Geometry check sheet. Reference: the model listing, model coordinates, mm. A direction names the side the tool comes from. Coordinates: 2 decimals unless noted, no trailing zeros. Write each loop counter-clockwise with the first axis right and the second up, starting at its lowest first coordinate (ties: lowest second). Pieces come first, ordered by that corner, then holes.
Autodesk Inventor part; units mm, degrees
ref_plane "Start plane" through (0, 0, 0) normal (0, 0, 1) x (1, 0, 0)
ref_plane "End plane" through (0, 0, 1263.65) normal (0, 0, 1) x (1, 0, 0)
ref_plane "Work Plane4" through (19.05, 0, 1263.65) normal (0, 0.7071, 0.7071) x (1, 0, 0)
ref_plane "Start plane" through (0, 0, 0) normal (0, 0, 1) x (1, 0, 0)
ref_plane "End plane" through (0, 0, 1263.65) normal (0, 0, 1) x (1, 0, 0)
sketch "Sketch" plane through (0, 0, 0) normal (0, 0, 1) x (1, 0, 0)
  line L0 (38.1, 0) -> (0, 0)
  line L1 (0, 0) -> (0, 38.1)
  line L2 (0, 38.1) -> (2.4765, 38.1)
  line L3 (4.7625, 35.814) -> (4.7625, 9.5885)
  line L4 (9.5885, 4.7625) -> (35.814, 4.7625)
  line L5 (38.1, 2.4765) -> (38.1, 0)
  line L6 (0, -11.0414) -> (0, 31.5385) construction
  line L7 (-11.0414, 0) -> (31.5385, 0) construction
  arc A0 (4.7625, 9.5885) -> (9.5885, 4.7625) centre (9.5885, 9.5885) ccw
  arc A1 (4.7625, 35.814) -> (2.4765, 38.1) centre (2.4765, 35.814) ccw
  arc A2 (38.1, 2.4765) -> (35.814, 4.7625) centre (35.814, 2.4765) ccw
  line L8 (0, 48.4964) -> (0, -20.9644) construction
  line L9 (-20.9644, 0) -> (48.4964, 0) construction
  point P0 (4.7625, 38.1)
  point P1 (4.7625, 4.7625)
  point P2 (38.1, 4.7625)
  dimension "d0" = 38.1
  dimension "d1" = 38.1
  dimension "d2" = 4.7625
  dimension "d3" = 4.7625
  dimension "d10" = 0
  dimension "d11" = 0
  dimension "d14" = 4.826
  dimension "d15" = 2.286
extrude "Body" add sketch "Sketch" along normal up to surface (1263.65 mm away) from surface at 0
sketch "Sketch3" plane through (0, 0, 0) normal (0, 0, 1) x (1, 0, 0)
  line L0 (0, 0) -> (10, 0)
ref_plane "Work Plane3" through (0, 0, 0) normal (0, -1, 0) x (1, 0, 0)
sketch "Sketch4" plane through (0, 0, 0) normal (0, -1, 0) x (1, 0, 0)
  line L0 (-2, 0) -> (12, 0)
  line L1 (-2, 1263.65) -> (12, 1263.65)
  dimension "d17" = 1263.65
ref_plane "Work Plane4" through (19.05, 0, 1263.65) normal (0, 0.7071, 0.7071) x (1, 0, 0)
split "Split1" plane through (19.05, 0, 1263.65) removes the side toward (0, 0.7071, 0.7071)
ref_plane "Work Plane5" through (19.05, 0, 0) normal (0, 0.7071, -0.7071) x (1, 0, 0)
split "Split2" plane through (19.05, 0, 0) removes the side toward (0, 0.7071, -0.7071)
equation "\"d0\" = G_H"
equation "\"d1\" = G_H"
equation "\"d2\" = G_T"
equation "\"d3\" = G_T"
equation "\"d14\" = G_IR"
equation "\"d15\" = G_ER"
equation "\"d4\" = G_L"
equation "\"G_H\" = 38.1"
equation "\"G_T\" = 4.7625"
equation "\"G_ER\" = 2.286"
equation "\"G_IR\" = 4.826"
equation "\"G_L\" = d17"
equation "\"ex\" = 0"
equation "\"G_OFFSET_START\" = 0"
equation "\"G_OFFSET_END\" = 0"
equation "\"d13\" = G_OFFSET_END + B_L"
equation "\"B_L\" = 1263.65"
properties part number "AISC - L 1.5 x 1.5 x 3/16 - 49.75" material "Steel, Mild"
1. Access from +Z, -Z, +X, -X, +Y, -Y to the whole of each face (thin tool, end or side, straight path). Record for faces 1 (the flat face through (0, 19, 623)), 2 (the flat face through (23, 4.762, 623)).
Computed values:
face 1: +Z, -Z, -X, +Y, -Y
face 2: +Z, -Z, +X, +Y
2. Sectioned sample at A-A, the plane z = 183.5. Record the boundary of the cut face in (x, y), and give its area (3 significant figures).
Computed values:
outline: (0, 0) - (38.1, 0) - (38.1, 2.48) arc R2.29 ccw to (35.81, 4.76) - (9.59, 4.76) arc R4.83 cw to (4.76, 9.59) - (4.76, 35.81) arc R2.29 ccw to (2.48, 38.1) - (0, 38.1) - close
area: 343 mm2
3. Sectioned sample at C-C, the plane x = 15.5. Record the boundary of the cut face in (y, z), and give its area (3 significant figures).
Computed values:
outline: (0, 0) - (4.76, 4.76) - (4.76, 1258.89) - (0, 1263.65) - close
area: 6,000 mm2
4. Gauge pin test, flat ends, axial feed: pin 1 Ø3 at (x, z) = (17.5, 716.5) entering from -Y; pin 2 Ø8 at (y, z) = (23.5, 480) entering from +X; pin 3 Ø8 at (x, y) = (23.5, 4.5) entering from -Z; pin 4 Ø21 at (x, z) = (24.5, 737) entering from +Y. Record the tip position at first contact, or that the pin passes through.
Computed values:
pin 1: stops at y = 0
pin 2: stops at x = 4.76
pin 3: stops at z = 0.5
pin 4: stops at y = 4.76
5. Thickness scan on line 1 along X through (y, z) = (25, 1138); line 2 along X through (y, z) = (4.5, 182.5). Record the ranges inside material, lowest first.
Computed values:
line 1: x = 0 to 4.76
line 2: x = 0 to 36.88
6. Sectioned sample at B-B, the plane y = 18.5. Record the boundary of the cut face in (x, z).
Computed values:
outline: (0, 18.5) - (4.76, 18.5) - (4.76, 1245.15) - (0, 1245.15) - close
